```python
from build123d import *

# Parameters (mm, degrees)
PAD_DEPTH       = 10
SKETCH001_R     = 7
PAD001_DEPTH    = 12
SKETCH002_R     = 5.7
PAD002_DEPTH    = 15
PAD003_DEPTH    = 34
SKETCH004_R     = 1.8
POCKET_DEPTH    = 11.5
SKETCH005_R     = 1.2
POCKET001_DEPTH = 18
SKETCH006_R     = 3.1
POCKET002_DEPTH = 4
CHAMFER_SIZE    = 12
FILLET_R        = 9


with BuildPart() as part:
    # Sketch → Pad (new body)
    with BuildSketch(Plane.XY):
        Polygon((-50, 0), (50, 0), (50, 57), (30, 57), (30, 25), (-30, 25), (-30, 57), (-50, 57), align=None)
    extrude(amount=PAD_DEPTH)

    # Sketch001 (on Face10 of Pad) → Pad001 (join)
    with BuildSketch(Plane.XY.offset(10)):
        with Locations((-40, 47)):
            Circle(SKETCH001_R)
        with Locations((40, 47)):
            Circle(SKETCH001_R)
    extrude(amount=PAD001_DEPTH)

    # Sketch002 (on Face14 of Pad001) → Pad002 (join)
    with BuildSketch(Plane.XY.offset(22)):
        with Locations((-40, 47)):
            Circle(SKETCH002_R)
        with Locations((40, 47)):
            Circle(SKETCH002_R)
    extrude(amount=PAD002_DEPTH)

    # Sketch003 (on Face5 of Pad002) → Pad003 (join)
    with BuildSketch(Plane.XY.offset(10)):
        Polygon((-50, 15), (-45.35, 15), (-45.35, 11.5), (-34.65, 11.5), (-34.65, 15), (34.65, 15), (34.65, 11.5), (45.35, 11.5), (45.35, 15), (50, 15), (50, 0), (-50, 0), align=None)
    extrude(amount=PAD003_DEPTH)

    # Sketch004 (on Face17 of Pad003) → Pocket (cut)
    with BuildSketch(Plane(origin=(0, 11.5, 0), x_dir=(-1, 0, 0), z_dir=(0, 1, 0))):
        with Locations((-40, 40)):
            Circle(SKETCH004_R)
        with Locations((-40, 21)):
            Circle(SKETCH004_R)
        with Locations((40, 40)):
            Circle(SKETCH004_R)
        with Locations((40, 21)):
            Circle(SKETCH004_R)
    extrude(amount=-POCKET_DEPTH, mode=Mode.SUBTRACT)

    # Sketch005 (on Face4 of Pocket) → Pocket001 (cut)
    with BuildSketch(Plane(origin=(0, 57, 0), x_dir=(-1, 0, 0), z_dir=(0, 1, 0))):
        with Locations((-40, 34.96648)):
            Circle(SKETCH005_R)
        with Locations((40, 34.96648)):
            Circle(SKETCH005_R)
    extrude(amount=-POCKET001_DEPTH, mode=Mode.SUBTRACT)

    # Sketch006 (on Face10 of Pocket001) → Pocket002 (cut)
    with BuildSketch(Plane.XZ):
        with Locations((-40, 40)):
            Circle(SKETCH006_R)
        with Locations((40, 40)):
            Circle(SKETCH006_R)
        with Locations((40, 21)):
            Circle(SKETCH006_R)
        with Locations((-40, 21)):
            Circle(SKETCH006_R)
    extrude(amount=-POCKET002_DEPTH, mode=Mode.SUBTRACT)

    # Chamfer
    chamfer_edges = [part.edges().sort_by_distance(p)[0] for p in [
        (-30, 25, 5),
        (30, 25, 5),
    ]]
    chamfer(chamfer_edges, length=CHAMFER_SIZE)

    # Fillet
    fillet_edges = [part.edges().sort_by_distance(p)[0] for p in [
        (-50, 57, 5),
        (-30, 57, 5),
        (30, 57, 5),
        (50, 57, 5),
    ]]
    fillet(fillet_edges, radius=FILLET_R)


solid = part.part
```
CAD build for the part. Positions are in the model's coordinates, mm. A direction names the side the tool comes from. Round coordinates to 2 decimals unless told otherwise and drop trailing zeros. Order: outer loops, then holes, each group sorted by start corner. A loop starts at its lowest first (then second) coordinate and runs counter-clockwise, first axis right, second up.
Q1. Wall check: L1, parallel to Z at x = 40, y = 6.25; L2, parallel to X at y = 42, z = 8; L3, parallel to Y at x = 17, z = 7. Give the ranges that are in metal, low to high.
Q2. Which spindle directions (+Z, -Z, +X, -X, +Y, -Y) get a long thin tool onto all of the face, cutting with end or side? Do faces 4 (the flat face through (34.65, 13, 27)), 5 (the flat face through (0, 25, 5)), 6 (the cylindrical face through (39.596, 1.972, 43.074)), 7 (the flat face through (-48, 15, 27)). Say none if no direction does.
Q3. Slice it at C-C (x = -40). State how many separate pieces and enclosed holes the cut face has, and give its area (3 significant figures).
Q4. Slice it at A-A (z = 40). Write the cut outline in (x, y), and give its area (3 significant figures).
Q5. Slice it at B-B (y = 31.5). Write the cut outline in (x, z), and give its area (3 significant figures).
Q6. Slice it at D-D (y = 47). Write the cut outline in (x, z), and give its area (3 significant figures).
Q7. Two-plate mould, pull along X, no slides. Class faces 1 (the flat face through (-40, 47, 37)), 2 (the flat face through (50, 13, 17)), 3 (the cylindrical face through (38.764, 41.436, 29.395)): pulls with the +X half, pulls with the -X half, needs draft (parallel to the pull), parting line crosses it, or undercut.
Q8. Drop flat-ended pins along their axis: pin 1 (6 mm diameter, centred on x = 38.5, z = 20, fed in from -Y); pin 2 (5.5 mm diameter, centred on x = -38.5, z = 28.5, fed in from +Y); pin 3 (3 mm diameter, centred on x = 33.5, z = 24, fed in from +Y); pin 4 (3 mm diameter, centred on x = -40, z = 21, fed in from +Y). Give the stop position or say it passes through.
Results below:
1. L1: z = 0 to 19.2, 22.8 to 38.2, 41.8 to 44
1. L2: x = -50 to -30, 30 to 50
1. L3: y = 0 to 25
2. face 4: +Z
2. face 5: +Z, -Z, +Y
2. face 6: -Y
2. face 7: +Z, +X, -X
3. separate pieces: 4
3. enclosed holes: 0
3. area: 1,170 mm2
4. outline: (-50, 0) - (-43.1, 0) - (-43.1, 4) - (-41.8, 4) - (-41.8, 11.5) - (-45.35, 11.5) - (-45.35, 15) - (-50, 15) - close; (-38.2, 4) - (-36.9, 4) - (-36.9, 0) - (36.9, 0) - (36.9, 4) - (38.2, 4) - (38.2, 11.5) - (34.65, 11.5) - (34.65, 15) - (-34.65, 15) - (-34.65, 11.5) - (-38.2, 11.5) - close; (41.8, 4) - (43.1, 4) - (43.1, 0) - (50, 0) - (50, 15) - (45.35, 15) - (45.35, 11.5) - (41.8, 11.5) - close
4. area: 1,320 mm2
5. outline: (-50, 0) - (-24.5, 0) - (-24.5, 10) - (-50, 10) - close; (24.5, 0) - (50, 0) - (50, 10) - (24.5, 10) - close
5. area: 510 mm2
6. outline: (-50, 0) - (-30, 0) - (-30, 10) - (-33, 10) - (-33, 22) - (-34.3, 22) - (-34.3, 37) - (-45.7, 37) - (-45.7, 22) - (-47, 22) - (-47, 10) - (-50, 10) - close; (30, 0) - (50, 0) - (50, 10) - (47, 10) - (47, 22) - (45.7, 22) - (45.7, 37) - (34.3, 37) - (34.3, 22) - (33, 22) - (33, 10) - (30, 10) - close; hole circle Ø2.4 at (-40, 34.97); hole circle Ø2.4 at (40, 34.97)
6. area: 1,070 mm2
7. face 1: needs draft
7. face 2: pulls with the +X half
7. face 3: undercut
8. pin 1: stops at y = 0
8. pin 2: stops at y = 52.7
8. pin 3: stops at y = 49.74
8. pin 4: stops at y = 54
